Check sheet for the drawn part. Datum: minimum x, y, z corner. Units: mm. Coordinates: 2 decimals unless noted, no trailing zeros. Write each loop counter-clockwise with the first axis right and the second up, starting at its lowest first coordinate (ties: lowest second). Pieces come first, ordered by that corner, then holes. Notation, with made-up numbers: (72.5, 14) -> (101.5, 14) arc R31 cw to (101.5, 53) -> close; hole circle Ø8 at (62.5, 13.25). An arc over 180 degrees is marked (long way). Write each question's results on one line, items separated by ' | '. Start each with the question number.
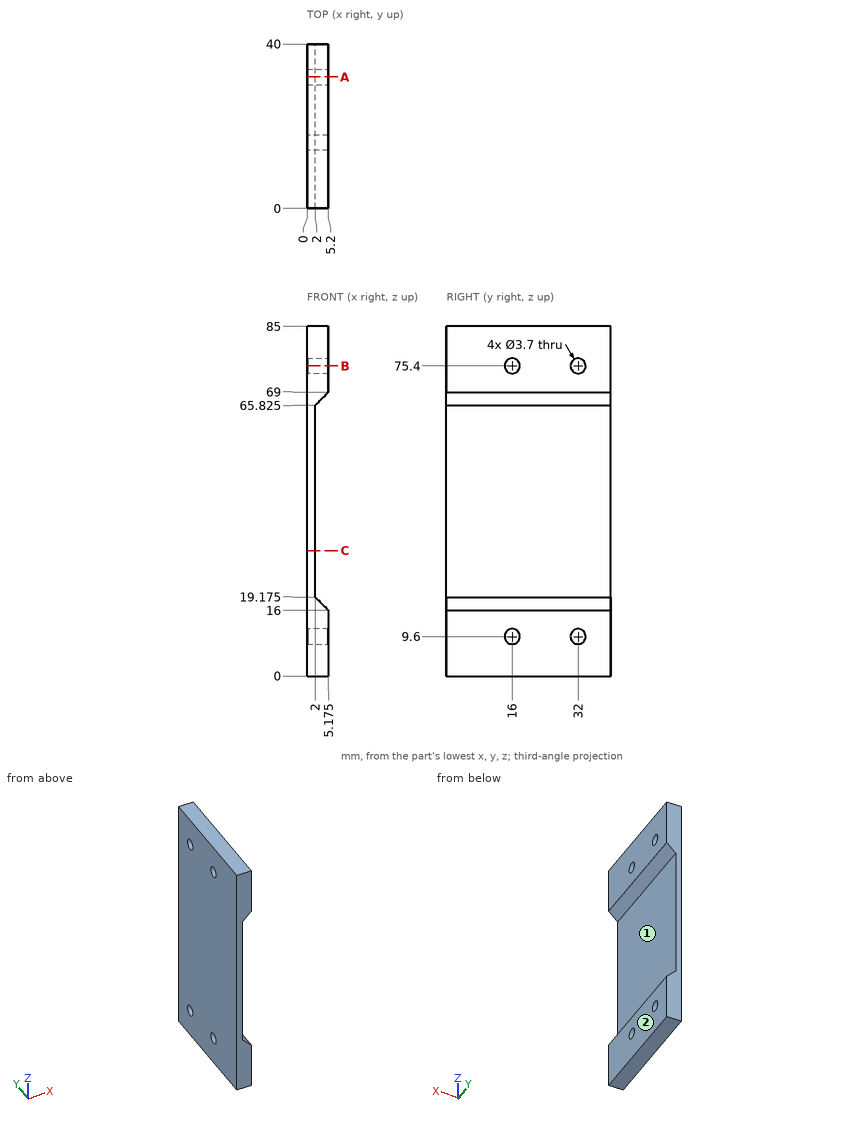
1. Sectioned sample at C-C on z = 30.5. Record the cut outline in (x, y), plus the area to 3 significant figures.
2. Depth check by flat-ended pin: pin 1 Ø1 at (x, y) = (3.5, 20.5) entering from -Z; pin 2 Ø12 at (y, z) = (22.5, 40.5) entering from +X. Enter the tip coordinate at first touch or a pass-through.
3. Sectioned sample at A-A on y = 32. Record the cut outline in (x, z) (3 decimals), plus the area to 3 significant figures.
4. Sectioned sample at B-B on z = 75.4. Record the cut outline in (x, y), plus the area to 3 significant figures.
5. Mould release check, pull along Z, two halves, no side actions. Record for the marked faces 1 and 2: +Z half, -Z half, draft (parallel to the pull), parting line (faces both ways), or undercut.
6. Material ranges on probe 1 along Y at (x, z) = (2.95, 75.4); probe 2 along Z at (x, y) = (0.8, 17); probe 3 along Y at (x, z) = (3.4, 8.5), recorded low to high. Write a range as from..to.
Computed values:
1) outline: (0, 0) -> (2, 0) -> (2, 40) -> (0, 40) -> close | area: 80.0 mm^2
2) pin 1: stops at z = 0 | pin 2: stops at x = 2
3) outline: (0, 0) -> (5.2, 0) -> (5.2, 7.75) -> (0, 7.75) -> close; (0, 11.45) -> (5.2, 11.45) -> (5.2, 16) -> (5.175, 16) -> (2, 19.175) -> (2, 65.825) -> (5.175, 69) -> (5.2, 69) -> (5.2, 73.55) -> (0, 73.55) -> close; (0, 77.25) -> (5.2, 77.25) -> (5.2, 85) -> (0, 85) -> close | area: 244 mm^2
4) outline: (0, 0) -> (5.2, 0) -> (5.2, 14.15) -> (0, 14.15) -> close; (0, 17.85) -> (5.2, 17.85) -> (5.2, 30.15) -> (0, 30.15) -> close; (0, 33.85) -> (5.2, 33.85) -> (5.2, 40) -> (0, 40) -> close | area: 170 mm^2
5) face 1: undercut | face 2: draft
6) probe 1: y = 0..14.15, 17.85..30.15, 33.85..40 | probe 2: z = 0..8.04, 11.16..73.84, 76.96..85 | probe 3: y = 0..14.51, 17.49..30.51, 33.49..40
